from build123d import *

# Parameters (mm, degrees)
REVOLVE1_ANGLE      = 180
BOSS_EXTRUDE3_DEPTH = 5
BOSS_EXTRUDE4_DEPTH = 5
SKETCH17_R          = 3.2385
CUT_EXTRUDE1_DEPTH  = 34
SKETCH18_R          = 4.75
CUT_EXTRUDE2_DEPTH  = 1.5
CHAMFER1_SIZE       = 0.5


with BuildPart() as part:
    # Sketch1 → Revolve1 (revolve)
    with BuildSketch(Plane.XY):
        Polygon((15, 26), (15, 26.75), (18, 25), (20, 25), (20, 33), (0, 33), (0, 26), align=None)
    revolve(axis=Axis((0, 0, 0), (1, 0, 0)), revolution_arc=REVOLVE1_ANGLE)

    # Sketch9 → Boss-Extrude3 (add)
    with BuildSketch(Plane(origin=(0, 0, 0), x_dir=(-1, 0, 0), z_dir=(0, 0, -1))):
        with BuildLine():
            Line((-20, 29), (0, 29))
            Line((0, 29), (0, 38))
            ThreePointArc((0, 38), (-10, 48), (-20, 38))
            Line((-20, 38), (-20, 29))
        make_face()
    extrude(amount=-BOSS_EXTRUDE3_DEPTH)

    # Sketch11 → Boss-Extrude4 (add)
    with BuildSketch(Plane(origin=(0, 0, 0), x_dir=(-1, 0, 0), z_dir=(0, 0, -1))):
        with BuildLine():
            Line((-20, -29), (0, -29))
            Line((0, -29), (0, -38))
            ThreePointArc((0, -38), (-10, -48), (-20, -38))
            Line((-20, -38), (-20, -29))
        make_face()
    extrude(amount=-BOSS_EXTRUDE4_DEPTH)

    # Sketch17 → Cut-Extrude1 (cut, through all)
    with BuildSketch(Plane(origin=(0, 0, 0), x_dir=(-1, 0, 0), z_dir=(0, 0, -1))):
        with Locations((-10, 38)):
            Circle(SKETCH17_R)
        with Locations((-10, -38)):
            Circle(SKETCH17_R)
    extrude(amount=-CUT_EXTRUDE1_DEPTH, mode=Mode.SUBTRACT)

    # Sketch18 → Cut-Extrude2 (cut)
    with BuildSketch(Plane.XY.offset(5)):
        with Locations((10, -38)):
            Circle(SKETCH18_R)
        with Locations((10, 38)):
            Circle(SKETCH18_R)
    extrude(amount=-CUT_EXTRUDE2_DEPTH, mode=Mode.SUBTRACT)

    # Chamfer1
    chamfer1_edges = [part.edges().sort_by_distance(p)[0] for p in [
        (20, 0, 25),
    ]]
    chamfer(chamfer1_edges, length=CHAMFER1_SIZE)


solid = part.part
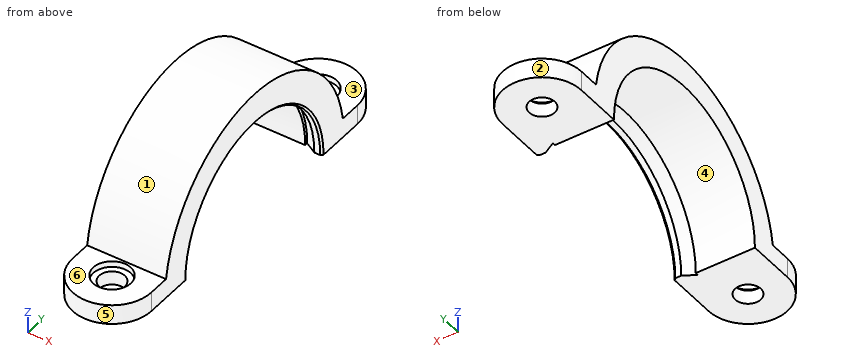
Design review of the part built by this model. Coordinates are the model's own, in mm. Face numbers are marked on the shaded views. A direction names the side the tool comes from. Round coordinates to 2 decimals unless told otherwise and drop trailing zeros. Write each loop counter-clockwise with the first axis right and the second up, starting at its lowest first coordinate (ties: lowest second). Pieces come first, ordered by that corner, then holes. Notation, with made-up numbers: (36, 86) -> (67, 86) arc R9 cw to (67, 98) -> close; hole circle Ø3 at (50.5, 28.25). An arc over 180 degrees is marked (long way). One line per item, written item: value. Start each with the question number.
Q1. Tool access review of the marked faces 5 and 6: name each direction out of +Z, -Z, +X, -X, +Y, -Y from which nothing blocks a thin tool from reaching the whole face with its end or side.
Q2. Add section C-C (x = 2). Give the boundary of the cut face in (y, z), then the cut area to 3 significant figures.
Q3. Insertion check: P1, Ø7.5, axis at x = 10, y = 38, coming from the -Z side; P2, Ø4.5, axis at x = 12.5, y = 41.5, coming from the +Z side; P3, Ø3, axis at x = 12.5, y = 36.5, coming from the +Z side; P4, Ø2, axis at x = 8.5, z = 14.5, coming from the -Y side. Each pin has a flat end and moves straight along its axis. Give the tip position at first contact, or say it passes through.
Q4. The part is to be moulded in two halves that separate along Y. For the marked faces 1, 2, 3 and 4, say which applies: pulls with the +Y half, pulls with the -Y half, needs draft (parallel to the pull), parting line crosses it, or undercut.
Q5. Add section B-B (y = 0). Give the boundary of the cut face in (x, z), then the cut area to 3 significant figures.
Q6. To check wall thickness, follow probe 1 along Y at (x, z) = (10, 0.9); probe 2 along Y at (x, z) = (10, 4.1); probe 3 along Y at (x, z) = (5.5, 20.5). State the ranges of each line that lie inside material, in increasing order.
Q7. Add section A-A (x = 10). Give the boundary of the cut face in (y, z), then the cut area to 3 significant figures.
Response:
1. face 5: +Z, -Z, -Y
1. face 6: +Z, +X, -X, -Y
2. outline: (-44, 0) -> (-26, 0) arc R26 cw to (26, 0) -> (44, 0) -> (44, 5) -> (32.62, 5) arc R33 ccw to (-32.62, 5) -> (-44, 5) -> close
2. area: 760 mm^2
3. P1: stops at z = 0
3. P2: stops at z = 5
3. P3: stops at z = 3.5
3. P4: stops at y = -30.11
4. face 1: parting line crosses it
4. face 2: pulls with the +Y half
4. face 3: needs draft
4. face 4: undercut
5. outline: (0, 26) -> (15, 26) -> (15, 26.75) -> (18, 25) -> (19.5, 25) -> (20, 25.5) -> (20, 33) -> (0, 33) -> close
5. area: 142 mm^2
6. probe 1: y = -48 to -41.24, -34.76 to -25.98, 25.98 to 34.76, 41.24 to 48
6. probe 2: y = -48 to -42.75, -33.25 to -25.67, 25.67 to 33.25, 42.75 to 48
6. probe 3: y = -25.86 to -15.99, 15.99 to 25.86
7. outline: (-48, 0) -> (-41.24, 0) -> (-41.24, 3.5) -> (-42.75, 3.5) -> (-42.75, 5) -> (-48, 5) -> close; (-34.76, 0) -> (-26, 0) arc R26 cw to (26, 0) -> (34.76, 0) -> (34.76, 3.5) -> (33.25, 3.5) -> (33.25, 5) -> (32.62, 5) arc R33 ccw to (-32.62, 5) -> (-33.25, 5) -> (-33.25, 3.5) -> (-34.76, 3.5) -> close; (41.24, 0) -> (48, 0) -> (48, 5) -> (42.75, 5) -> (42.75, 3.5) -> (41.24, 3.5) -> close
7. area: 726 mm^2
